Could you check a few things on this model? Use its own coordinates, in mm. Face numbers are marked on the shaded views. A direction names the side the tool comes from. Give positions to 0.01 mm unless a question says otherwise; leave off trailing zeros. Write each loop counter-clockwise with the first axis right and the second up, starting at its lowest first coordinate (ties: lowest second). Pieces come first, ordered by that corner, then holes. Notation, with made-up numbers: (-5, 51) -> (14, 51) arc R30 ccw to (14, 84) -> close; hole circle Ø5 at (-5.5, 35). An arc over 180 degrees is marked (long way). One line per question, with ' | ' between items.
from build123d import *

# Parameters (mm, degrees)
BOSS_EXTRUDE1_DEPTH            = 10
BOSS_EXTRUDE1_DEPTH_BACK       = 10
FILLET1_R                      = 1
BOSS_EXTRUDE2_START            = -10
BOSS_EXTRUDE2_DEPTH            = 20
FILLET2_R                      = 5
BOSS_EXTRUDE3_DEPTH            = 4
BOSS_EXTRUDE3_DEPTH_BACK       = 9
FILLET3_R                      = 1
FILLET4_R                      = 2
CUT_EXTRUDE1_REACH             = 35.208
SKETCH4_R                      = 1.5
CUT_EXTRUDE2_REACH             = 38.208
SKETCH5_R                      = 1.5
CUT_EXTRUDE2_DIRECTION_2_REACH = 38.208
FILLET5_R                      = 2


with BuildPart() as part:
    # Sketch1 → Boss-Extrude1 (new, two sides: drawn at the far end of the back side and taken through both)
    with BuildSketch(Plane(origin=(0, 0, 0), x_dir=(0, 0, -1), z_dir=(1, 0, 0)).offset(-BOSS_EXTRUDE1_DEPTH_BACK)):
        with BuildLine():
            Line((-5.175905718, 0.5), (-14.791561976, 0.5))
            Line((-14.791561976, 0.5), (-14.791561976, 3.5))
            Line((-14.791561976, 3.5), (-8.291561976, 3.5))
            ThreePointArc((-8.291561976, 3.5), (9, 0), (-8.291561976, -3.5))
            Line((-8.291561976, -3.5), (-14.791561976, -3.5))
            Line((-14.791561976, -3.5), (-14.791561976, -0.5))
            Line((-14.791561976, -0.5), (-5.175905718, -0.5))
            ThreePointArc((-5.175905718, -0.5), (5.2, 0), (-5.175905718, 0.5))
        make_face()
    extrude(amount=BOSS_EXTRUDE1_DEPTH + BOSS_EXTRUDE1_DEPTH_BACK)

    # Fillet1
    fillet1_edges = [part.edges().sort_by_distance(p)[0] for p in [
        (0, 3.5, 8.291561976),
        (0, -3.5, 8.291561976),
    ]]
    fillet(fillet1_edges, radius=FILLET1_R)

    # Sketch2 → Boss-Extrude2 (add)
    with BuildSketch(Plane(origin=(0, 0, 0), x_dir=(0, 0, -1), z_dir=(1, 0, 0)).offset(BOSS_EXTRUDE2_START)):
        with BuildLine():
            Line((-4, 8.062257748), (-4, 9.5))
            Line((-4, 9.5), (4, 9.5))
            Line((4, 9.5), (9, 9.5))
            Line((9, 9.5), (9, 0))
            ThreePointArc((9, 0), (7.64852927, 4.74341649), (4, 8.062257748))
            Line((4, 8.062257748), (-4, 8.062257748))
        make_face()
    extrude(amount=BOSS_EXTRUDE2_DEPTH)

    # Fillet2
    # the kernel refuses this fillet: 5 mm, written as the material it adds along each edge
    with BuildSketch(Plane(origin=(-10, 8.062257748, 4), x_dir=(0, -0.5399133181781692, 0.8417206239922121), z_dir=(1, 0, 0))) as fillet2_piece_1:
        with BuildLine():
            CenterArc((2.519874472, -4.969901053), FILLET2_R, 96.289938273, 34.950941651)
            Line((-0.77625619, -1.210177305), (-0.842178803, -1.13498283))
            ThreePointArc((-0.842178803, -1.13498283), (-0.472300157, -0.551097321), (-0.084172062, 0.053991332))
            Line((-0.084172062, 0.053991332), (0.010955976, 0.099398021))
            ThreePointArc((0.010955976, 0.099398021), (0.986037837, 0.045821895), (1.961119698, 0.099398021))
            Line((1.961119698, 0.099398021), (1.972075674, 0))
        make_face()
    extrude(amount=20)

    # Sketch3 → Boss-Extrude3 (add, two sides: drawn at the far end of the back side and taken through both)
    with BuildSketch(Plane.XY.offset(-BOSS_EXTRUDE3_DEPTH_BACK)):
        Polygon((-5.2, 9.5), (-5.2, 19.9), (-0.5, 19.9), (-0.5, 31.5), (-3.5, 31.5), (-3.5, 23), (-10, 23), (-10, 9.5), align=None)
        Polygon((5.2, 19.9), (5.2, 9.5), (10, 9.5), (10, 23), (3.5, 23), (3.5, 31.5), (0.5, 31.5), (0.5, 19.9), align=None)
    extrude(amount=BOSS_EXTRUDE3_DEPTH + BOSS_EXTRUDE3_DEPTH_BACK)

    # Fillet3
    fillet3_edges = [part.edges().sort_by_distance(p)[0] for p in [
        (-5.2, 9.5, -2.5),
        (-5.2, 19.9, -2.5),
        (5.2, 19.9, -2.5),
        (5.2, 9.5, -2.5),
    ]]
    fillet(fillet3_edges, radius=FILLET3_R)

    # Fillet4
    fillet4_edges = [part.edges().sort_by_distance(p)[0] for p in [
        (-3.5, 23, -2.5),
        (-10, 23, -2.5),
        (10, 23, -2.5),
        (3.5, 23, -2.5),
    ]]
    fillet(fillet4_edges, radius=FILLET4_R)

    # Cut-Extrude1: up to this face of the body (flat: up to its plane)
    cut_extrude1_end = Plane(part.part.faces().sort_by_distance((0, -3.5, 11.860923763))[0])
    # Sketch4 → Cut-Extrude1 (cut, up to the picked face)
    with BuildSketch(Plane(origin=(0, 3.5, 0), x_dir=(1, 0, 0), z_dir=(0, 1, 0)), mode=Mode.PRIVATE) as cut_extrude1_sk1:
        with Locations(Location((-5, -11.860923763, 0), (0, 0, 270))):
            Circle(SKETCH4_R)
    cut_extrude1_tool1 = split(extrude(cut_extrude1_sk1.sketch, amount=-CUT_EXTRUDE1_REACH, mode=Mode.PRIVATE), bisect_by=cut_extrude1_end, keep=Keep.BOTH, mode=Mode.PRIVATE)
    # Sketch4 → Cut-Extrude1 (cut, up to the picked face)
    with BuildSketch(Plane(origin=(0, 3.5, 0), x_dir=(1, 0, 0), z_dir=(0, 1, 0)), mode=Mode.PRIVATE) as cut_extrude1_sk2:
        with Locations(Location((5, -11.860923763, 0), (0, 0, 270))):
            Circle(SKETCH4_R)
    cut_extrude1_tool2 = split(extrude(cut_extrude1_sk2.sketch, amount=-CUT_EXTRUDE1_REACH, mode=Mode.PRIVATE), bisect_by=cut_extrude1_end, keep=Keep.BOTH, mode=Mode.PRIVATE)
    add(cut_extrude1_tool1.solids().sort_by(Axis((-5, 3.5, 11.860924), (0, -1, 0)))[0], mode=Mode.SUBTRACT)
    add(cut_extrude1_tool2.solids().sort_by(Axis((5, 3.5, 11.860924), (0, -1, 0)))[0], mode=Mode.SUBTRACT)

    # Cut-Extrude2: up to this face of the body (flat: up to its plane)
    cut_extrude2_end = Plane(part.part.faces().sort_by_distance((-3.5, 28.25, -2.5))[0])
    # Sketch5 → Cut-Extrude2 (cut, up to the picked face)
    with BuildSketch(Plane(origin=(0, 0, 0), x_dir=(0, 0, -1), z_dir=(1, 0, 0)), mode=Mode.PRIVATE) as cut_extrude2_sk1:
        with Locations((2.5, 28.25)):
            Circle(SKETCH5_R)
    cut_extrude2_tool1 = split(extrude(cut_extrude2_sk1.sketch, amount=-CUT_EXTRUDE2_REACH, mode=Mode.PRIVATE), bisect_by=cut_extrude2_end, keep=Keep.BOTH, mode=Mode.PRIVATE)
    add(cut_extrude2_tool1.solids().sort_by(Axis((0, 28.25, -2.5), (-1, 0, 0)))[0], mode=Mode.SUBTRACT)

    # Cut-Extrude2 direction 2: up to this face of the body (flat: up to its plane)
    cut_extrude2_direction_2_end = Plane(part.part.faces().sort_by_distance((3.5, 28.25, -2.5))[0])
    # Sketch5 → Cut-Extrude2 direction 2 (cut, up to the picked face)
    with BuildSketch(Plane(origin=(0, 0, 0), x_dir=(0, 0, -1), z_dir=(1, 0, 0)), mode=Mode.PRIVATE) as cut_extrude2_direction_2_sk1:
        with Locations((2.5, 28.25)):
            Circle(SKETCH5_R)
    cut_extrude2_direction_2_tool1 = split(extrude(cut_extrude2_direction_2_sk1.sketch, amount=CUT_EXTRUDE2_DIRECTION_2_REACH, mode=Mode.PRIVATE), bisect_by=cut_extrude2_direction_2_end, keep=Keep.BOTH, mode=Mode.PRIVATE)
    add(cut_extrude2_direction_2_tool1.solids().sort_by(Axis((0, 28.25, -2.5), (1, 0, 0)))[0], mode=Mode.SUBTRACT)

    # Fillet5
    fillet5_edges = [part.edges().sort_by_distance(p)[0] for p in [
        (0, 0.5, 5.175905718),
        (0, -0.5, 5.175905718),
        (-0.5, 19.9, -2.5),
        (0.5, 19.9, -2.5),
    ]]
    fillet(fillet5_edges, radius=FILLET5_R)


solid = part.part
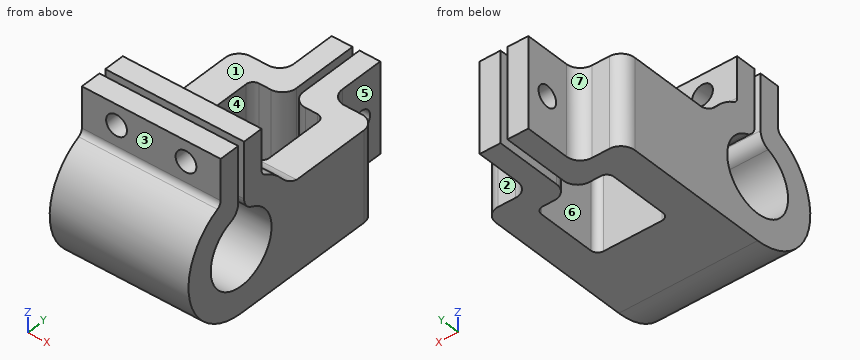
Q1. If I drill on line 1 along Y through (x, z) = (0.25, 9); line 2 along Y through (x, z) = (-5, -1.5); line 3 along Y through (x, z) = (2.75, -3), over which ranges is the centre line in solid material (lowest first)?
Answer below:
line 1: y = -3.5 to -0.5, 0.5 to 3.5 | line 2: y = -8.87 to -4.98, 4.98 to 9.9, 19.5 to 23.06 | line 3: y = -8.49 to -4.25, 4.25 to 9.5, 19.9 to 26.84, 29.66 to 31.5
Q2. Imagine slicing it at D-D on z = -2.5. Count the separate pieces of the cut face and the enclosed holes in it, and give its area (3 significant figures).
Answer below:
separate pieces: 4 | enclosed holes: 0 | area: 371 mm^2
Q3. Imagine slicing it at A-A on y = 28.25. Please give me the cut outline in (x, z), and give its area (3 significant figures).
Answer below:
outline: (-3.5, -9) -> (-0.5, -9) -> (-0.5, -4) -> (-3.5, -4) -> close; (-3.5, -1) -> (-0.5, -1) -> (-0.5, 4) -> (-3.5, 4) -> close; (0.5, -9) -> (3.5, -9) -> (3.5, -4) -> (0.5, -4) -> close; (0.5, -1) -> (3.5, -1) -> (3.5, 4) -> (0.5, 4) -> close | area: 60.0 mm^2
Q4. If we mould it in two halves opening along Y, with no side actions, what happens to the marked faces 5, 6 and 7? For each: +Y half, -Y half, draft (parallel to the pull), parting line (faces both ways), or undercut.
Answer below:
face 5: draft | face 6: undercut | face 7: +Y half
Q5. Imagine slicing it at B-B on y = 1. Please give me the cut outline in (x, z), and give its area (3 significant figures).
Answer below:
outline: (-10, -9) -> (10, -9) -> (10, -5.1) -> (-10, -5.1) -> close; (-10, 5.43) -> (10, 5.43) -> (10, 14.79) -> (-10, 14.79) -> close; hole circle Ø3 at (-5, 11.86); hole circle Ø3 at (5, 11.86) | area: 251 mm^2
Q6. Will these pins go through, and if not, where does the flat tip stop? pin 1 (2 mm diameter, centred on y = 29, z = -2, fed in from -X); pin 2 (0.9 mm diameter, centred on x = 3.5, z = -3, fed in from -Y); pin 3 (5 mm diameter, centred on y = 28.25, z = -2.5, fed in from +X).
Answer below:
pin 1: stops at x = -3.5 | pin 2: stops at y = -8.63 | pin 3: stops at x = 3.5
Q7. On a 3-axis mill with a long thin cutter (end or side, diameter ignored), from which of +Z, -Z, +X, -X, +Y, -Y can I reach the whole of each face in a straight line? I mean the marked faces 1, 2, 3 and 4. Say none if no direction works.
Answer below:
face 1: +Z, +X, -X, +Y | face 2: +Z, -Z, +X, +Y | face 3: +Z, +X, -X, -Y | face 4: +Z, -Z
